Geometry: final body of the model. Coordinates: model frame, mm. A direction names the side the tool comes from. Round coordinates to 2 decimals unless told otherwise and drop trailing zeros. Loops run counter-clockwise (first coordinate to the right, second up) from the corner with the lowest first, then second, coordinate; pieces in that order, holes last. Notation, with made-up numbers: (-26, -10) - (8, -10) arc R6 ccw to (8, 1) - close; hole circle Ø1 at (80.5, 10.5). An arc over 180 degrees is marked (long way). Answer as a JSON object with one key per item and string values. Group by question number.
Item 1: Line query: line 1 (X direction, y = -0.3, z = 7.7); line 2 (Z direction, x = -6.35, y = -0.65); line 3 (Y direction, x = 1.5, z = 1.5). Output: solid intervals per line, ascending.
Item 2: Reachability of faces 5 (the face through (-6.398, 1.327, 1.357)), 6 (the face through (2.03, -6, 11)), 7 (the face through (-13, -12.55, 8)) from +Z, -Z, +X, -X, +Y, -Y: full face, straight path, thin tool, end or side. Return the list, or none.
Item 3: Section B-B (x = -6.35). Return the cut outline in (y, z).
Item 4: Section A-A (z = 4). Return the cut outline in (x, y).
Item 5: Section C-C (y = -10.75). Return the cut outline in (x, z).
Item 6: Section D-D (z = 7.7). Return the cut outline in (x, y).
Item 7: First-contact query: pin 1 (7 mm diameter, centred on x = -7, y = -3.5, fed in from -Z); pin 2 (0.7 mm diameter, centred on x = -15.5, y = -5.5, fed in from +Z); pin 3 (3.5 mm diameter, centred on y = -3, z = 5.5, fed in from -X). Flat tips, straight axial feed; report the tip coordinate or a pass-through.
Item 8: Draft query along X for faces 1 (the face through (2.03, -6, 5)), 2 (the face through (-16.245, 1.123, 0.801)), 3 (the face through (-9.243, 1.245, 14.327)), 4 (the face through (-6, 0.95, 13)). Return one class per face: released by +X, released by -X, zero draft, split by the parting line, or undercut.
Autodesk Inventor part; units mm, degrees
ref_plane "Work Plane9" through (-1.05, -12.7, 2.7) normal (0, 1, 0) x (0, 0, 1)
ref_plane "YZ Plane" through (0, 0, 0) normal (1, 0, 0) x (0, 1, 0)
ref_plane "XZ Plane" through (0, 0, 0) normal (0, 1, 0) x (-1, 0, 0)
ref_plane "Work Plane8" through (7.15, 0.8, 25.4) normal (0, 1, 0) x (1, 0, 0)
sketch "Sketch21" plane through (7.15, 0.8, 25.4) normal (0, 1, 0) x (1, 0, 0)
  line L0 (-3, 3) -> (-24, 3)
  line L1 (-3, 197) -> (-3, 3)
  line L2 (-24, 197) -> (-3, 197)
  line L3 (-24, 3) -> (-24, 197)
  line L4 (-4.819988, 19.366667) -> (-3.319988, 19.366667)
  line L5 (-3.319988, 19.366667) -> (-3.319988, 16.033333)
  line L6 (-3.319988, 16.033333) -> (-4.819988, 16.033333)
  line L7 (-4.819988, 16.033333) -> (-4.819988, 12.7)
  line L8 (-4.819988, 12.7) -> (-22.180012, 12.7)
  line L9 (-22.180012, 12.7) -> (-22.180012, 16.033333)
  line L10 (-22.180012, 16.033333) -> (-23.680012, 16.033333)
  line L11 (-23.680012, 16.033333) -> (-23.680012, 19.366667)
  line L12 (-23.680012, 19.366667) -> (-22.180012, 19.366667)
  line L13 (-22.180012, 19.366667) -> (-22.180012, 22.7)
  line L14 (-22.180012, 22.7) -> (-4.819988, 22.7)
  line L15 (-4.819988, 22.7) -> (-4.819988, 19.366667)
  line L16 (-21.880012, 22.4) -> (-21.880012, 19.066667)
  line L17 (-21.880012, 19.066667) -> (-23.380012, 19.066667)
  line L18 (-23.380012, 19.066667) -> (-23.380012, 16.333333)
  line L19 (-23.380012, 16.333333) -> (-21.880012, 16.333333)
  line L20 (-21.880012, 16.333333) -> (-21.880012, 13)
  line L21 (-21.880012, 13) -> (-5.119988, 13)
  line L22 (-5.119988, 13) -> (-5.119988, 16.333333)
  line L23 (-5.119988, 16.333333) -> (-3.619988, 16.333333)
  line L24 (-3.619988, 16.333333) -> (-3.619988, 19.066667)
  line L25 (-3.619988, 19.066667) -> (-5.119988, 19.066667)
  line L26 (-5.119988, 19.066667) -> (-5.119988, 22.4)
  line L27 (-5.119988, 22.4) -> (-21.880012, 22.4)
  point P0 (-7.15, 25.4)
  dimension "d99" = 0.3
  dimension "d100" = 0.3
  dimension "d101" = 0.3
  dimension "d102" = 0.3
  dimension "d103" = 0.3
  dimension "d104" = 0.3
  dimension "d105" = 0.3
  dimension "d106" = 0.3
  dimension "d107" = 0.3
  dimension "d108" = 0.3
  dimension "d109" = 0.3
  dimension "d110" = 0.3
ref_plane "Work Plane9" through (-1.05, -12.7, 2.7) normal (0, 1, 0) x (0, 0, 1)
sketch "Sketch21 outline for Extrusion20" plane through (7.15, 0.8, 25.4) normal (0, 1, 0) x (1, 0, 0)
  line L0 (-5.119988, 22.4) -> (-21.880012, 22.4)
  line L1 (-5.119988, 19.066667) -> (-5.119988, 22.4)
  line L2 (-3.619988, 19.066667) -> (-5.119988, 19.066667)
  line L3 (-3.619988, 16.333333) -> (-3.619988, 19.066667)
  line L4 (-5.119988, 16.333333) -> (-3.619988, 16.333333)
  line L5 (-5.119988, 13) -> (-5.119988, 16.333333)
  line L6 (-21.880012, 13) -> (-5.119988, 13)
  line L7 (-21.880012, 16.333333) -> (-21.880012, 13)
  line L8 (-23.380012, 16.333333) -> (-21.880012, 16.333333)
  line L9 (-23.380012, 19.066667) -> (-23.380012, 16.333333)
  line L10 (-21.880012, 19.066667) -> (-23.380012, 19.066667)
  line L11 (-21.880012, 22.4) -> (-21.880012, 19.066667)
extrude "Extrusion20" add sketch "Sketch21 outline for Extrusion20" against normal up to surface (13.5 mm away)
sketch "Sketch22" plane through (-14.730012, 0.8, 12.4) normal (0, 0, 1) x (1, 0, 0)
  circle A0 centre (8.380012, -13.5) radius 5 construction
  arc A1 (3.080012, -13.5) -> (13.680012, -13.5) centre (8.380012, -13.5) ccw
  arc A2 (13.680012, -13.5) -> (3.080012, -13.5) centre (8.380012, -13.5) ccw
  point P0 (14.730012, -0.8)
sketch "Sketch22 outline for Extrusion21" plane through (-14.730012, 0.8, 12.4) normal (0, 0, 1) x (1, 0, 0)
  arc A0 (13.680012, -13.5) -> (3.080012, -13.5) centre (8.380012, -13.5) ccw
  arc A1 (3.080012, -13.5) -> (13.680012, -13.5) centre (8.380012, -13.5) ccw
extrude "Extrusion21" cut sketch "Sketch22 outline for Extrusion21" against normal through all
sketch "Sketch23" plane through (7.15, 0.8, 25.4) normal (0, 1, 0) x (1, 0, 0)
  line L0 (-21.880012, 22.4) -> (-21.880012, 19.066667)
  line L1 (-21.880012, 19.066667) -> (-23.380012, 19.066667)
  line L2 (-23.380012, 19.066667) -> (-23.380012, 16.333333)
  line L3 (-23.380012, 16.333333) -> (-21.880012, 16.333333)
  line L4 (-21.880012, 16.333333) -> (-21.880012, 13)
  line L5 (-21.880012, 13) -> (-5.119988, 13)
  line L6 (-5.119988, 13) -> (-5.119988, 16.333333)
  line L7 (-5.119988, 16.333333) -> (-3.619988, 16.333333)
  line L8 (-3.619988, 16.333333) -> (-3.619988, 19.066667)
  line L9 (-3.619988, 19.066667) -> (-5.119988, 19.066667)
  line L10 (-5.119988, 19.066667) -> (-5.119988, 22.4)
  line L11 (-5.119988, 22.4) -> (-21.880012, 22.4)
  line L12 (-24, 3) -> (-24, 197)
  line L13 (-3, 197) -> (-3, 3)
  line L14 (-23.680012, 24.9) -> (-3.319988, 24.9)
  line L15 (-3.319988, 24.9) -> (-3.319988, 10.5)
  line L16 (-3.319988, 10.5) -> (-23.680012, 10.5)
  line L17 (-23.680012, 10.5) -> (-23.680012, 24.9)
  point P0 (-7.15, 25.4)
  dimension "d115" = 2.5
  dimension "d116" = 2.5
  dimension "d117" = 0.3
  dimension "d118" = 0.3
sketch "Sketch23 outline for Extrusion22" plane through (7.15, 0.8, 25.4) normal (0, 1, 0) x (1, 0, 0)
  line L0 (-23.680012, 24.9) -> (-3.319988, 24.9)
  line L1 (-3.319988, 24.9) -> (-3.319988, 10.5)
  line L2 (-3.319988, 10.5) -> (-23.680012, 10.5)
  line L3 (-23.680012, 10.5) -> (-23.680012, 24.9)
extrude "Extrusion22" add sketch "Sketch23 outline for Extrusion22" along normal blind 1.5
sketch "Sketch24" plane through (-16.530012, 0.8, 14.9) normal (0, 0, 1) x (1, 0, 0)
  line L0 (20.360025, 1.5) -> (0, 1.5)
  line L1 (0, 0) -> (0, 1.5)
  line L2 (20.360025, 0) -> (0, 0)
  line L3 (20.360025, 0) -> (20.360025, 1.5)
  line L4 (6.786675, 0) -> (13.57335, 0)
  line L5 (13.57335, 0) -> (13.57335, 0.75)
  line L6 (13.57335, 0.75) -> (6.786675, 0.75)
  line L7 (6.786675, 0.75) -> (6.786675, 0)
  point P0 (16.530012, -0.8)
  dimension "d121" = 20.36002
  dimension "d122" = 6.78667
  dimension "d123" = 6.78667
  dimension "d124" = 0.75
  dimension "d125" = 1.5
sketch "Sketch24 outline for Extrusion23" plane through (-16.530012, 0.8, 14.9) normal (0, 0, 1) x (1, 0, 0)
  line L0 (6.786675, 0.75) -> (6.786675, 0)
  line L1 (13.57335, 0.75) -> (6.786675, 0.75)
  line L2 (13.57335, 0) -> (13.57335, 0.75)
  line L3 (6.786675, 0) -> (13.57335, 0)
extrude "Extrusion23" cut sketch "Sketch24 outline for Extrusion23" against normal blind 1.5
sketch "Sketch25" plane through (3.830012, 0.8, 0.5) normal (0, 0, -1) x (-1, 0, 0)
  line L0 (6.786675, 0.75) -> (6.786675, 0)
  line L1 (13.57335, 0.75) -> (6.786675, 0.75)
  line L2 (13.57335, 0) -> (13.57335, 0.75)
  line L3 (20.360025, 0) -> (0, 0)
  point P0 (3.830012, -0.8)
fillet "Fillet13" radius 2 3 edges at (-9.7433, 1.55, 14.15) (-2.9567, 1.55, 14.15) (-6.35, 1.55, 13.4)
sketch "Sketch25 outline for Extrusion24" plane through (3.830012, 0.8, 0.5) normal (0, 0, -1) x (-1, 0, 0)
  line L0 (13.57335, 0.75) -> (6.786675, 0.75)
  line L1 (13.57335, 0) -> (13.57335, 0.75)
  line L2 (6.786675, 0) -> (13.57335, 0)
  line L3 (6.786675, 0.75) -> (6.786675, 0)
extrude "Extrusion24" cut sketch "Sketch25 outline for Extrusion24" against normal blind 1.5
fillet "Fillet14" radius 2 3 edges at (-2.9567, 1.55, 1.25) (-9.7433, 1.55, 1.25) (-6.35, 1.55, 2)
fillet "Fillet15" radius 1 8 edges at (-6.35, 2.3, 0.5) (3.83, 2.3, 7.7) (-6.35, 2.3, 14.9) (-16.53, 2.3, 7.7) (3.83, 1.55, 0.5) (3.83, 1.55, 14.9) (-16.53, 1.55, 0.5) (-16.53, 1.55, 14.9)
sketch "Sketch26" plane through (-16.230012, -12.7, 9.066667) normal (0, -1, 0) x (1, 0, 0)
  line L0 (4.580012, -6.066667) -> (4.580012, 3.333333)
  line L1 (4.580012, 3.333333) -> (1.5, 3.333333)
  line L2 (1.5, 3.333333) -> (1.5, 0)
  line L3 (1.5, 0) -> (0, 0)
  line L4 (0, 0) -> (0, -2.733333)
  line L5 (0, -2.733333) -> (1.5, -2.733333)
  line L6 (1.5, -2.733333) -> (1.5, -6.066667)
  line L7 (1.5, -6.066667) -> (4.580012, -6.066667)
  line L8 (15.180012, 3.333333) -> (15.180012, -6.066667)
  line L9 (15.180012, -6.066667) -> (18.260025, -6.066667)
  line L10 (18.260025, -6.066667) -> (18.260025, -2.733333)
  line L11 (18.260025, -2.733333) -> (19.760025, -2.733333)
  line L12 (19.760025, -2.733333) -> (19.760025, 0)
  line L13 (19.760025, 0) -> (18.260025, 0)
  line L14 (18.260025, 0) -> (18.260025, 3.333333)
  line L15 (18.260025, 3.333333) -> (15.180012, 3.333333)
  point P0 (16.230012, -9.066667)
sketch "Sketch26 outline for Extrusion25" plane through (-16.230012, -12.7, 9.066667) normal (0, -1, 0) x (1, 0, 0)
  line L0 (1.5, -6.066667) -> (4.580012, -6.066667)
  line L1 (1.5, -2.733333) -> (1.5, -6.066667)
  line L2 (0, -2.733333) -> (1.5, -2.733333)
  line L3 (0, 0) -> (0, -2.733333)
  line L4 (1.5, 0) -> (0, 0)
  line L5 (1.5, 3.333333) -> (1.5, 0)
  line L6 (4.580012, 3.333333) -> (1.5, 3.333333)
  line L7 (4.580012, -6.066667) -> (4.580012, 3.333333)
  line L8 (18.260025, 3.333333) -> (15.180012, 3.333333)
  line L9 (18.260025, 0) -> (18.260025, 3.333333)
  line L10 (19.760025, 0) -> (18.260025, 0)
  line L11 (19.760025, -2.733333) -> (19.760025, 0)
  line L12 (18.260025, -2.733333) -> (19.760025, -2.733333)
  line L13 (18.260025, -6.066667) -> (18.260025, -2.733333)
  line L14 (15.180012, -6.066667) -> (18.260025, -6.066667)
  line L15 (15.180012, 3.333333) -> (15.180012, -6.066667)
extrude "Extrusion25" cut sketch "Sketch26 outline for Extrusion25" against normal blind 0.15
sketch "Sketch27" plane through (7.15, 0.8, 25.4) normal (0, -1, 0) x (1, 0, 0)
  line L0 (-3.619988, -16.333333) -> (-3.619988, -19.066667)
  line L1 (-3.619988, -19.066667) -> (-5.119988, -19.066667)
  line L2 (-5.119988, -19.066667) -> (-5.119988, -22.4)
  line L3 (-5.119988, -22.4) -> (-21.880012, -22.4)
  line L4 (-21.880012, -22.4) -> (-21.880012, -19.066667)
  line L5 (-21.880012, -19.066667) -> (-23.380012, -19.066667)
  line L6 (-23.380012, -19.066667) -> (-23.380012, -16.333333)
  line L7 (-23.380012, -16.333333) -> (-21.880012, -16.333333)
  line L8 (-21.880012, -16.333333) -> (-21.880012, -13)
  line L9 (-21.880012, -13) -> (-5.119988, -13)
  line L10 (-5.119988, -13) -> (-5.119988, -16.333333)
  line L11 (-5.119988, -16.333333) -> (-3.619988, -16.333333)
  arc A0 (-22.680012, -10.5) -> (-23.680012, -11.5) centre (-22.680012, -11.5) ccw
  line L12 (-23.680012, -11.5) -> (-23.680012, -23.9)
  arc A1 (-23.680012, -23.9) -> (-22.680012, -24.9) centre (-22.680012, -23.9) ccw
  line L13 (-22.680012, -24.9) -> (-16.893337, -24.9)
  line L14 (-16.893337, -24.9) -> (-16.893337, -23.4)
  line L15 (-16.893337, -23.4) -> (-10.106663, -23.4)
  line L16 (-10.106663, -23.4) -> (-10.106663, -24.9)
  line L17 (-10.106663, -24.9) -> (-4.319988, -24.9)
  arc A2 (-4.319988, -24.9) -> (-3.319988, -23.9) centre (-4.319988, -23.9) ccw
  line L18 (-3.319988, -23.9) -> (-3.319988, -11.5)
  arc A3 (-3.319988, -11.5) -> (-4.319988, -10.5) centre (-4.319988, -11.5) ccw
  line L19 (-4.319988, -10.5) -> (-10.106663, -10.5)
  line L20 (-10.106663, -10.5) -> (-10.106663, -12)
  line L21 (-10.106663, -12) -> (-16.893337, -12)
  line L22 (-16.893337, -12) -> (-16.893337, -10.5)
  line L23 (-16.893337, -10.5) -> (-22.680012, -10.5)
  point P0 (-7.15, -25.4)
sketch "Sketch27 outline for Extrusion26" plane through (7.15, 0.8, 25.4) normal (0, -1, 0) x (1, 0, 0)
  line L0 (-16.893337, -10.5) -> (-22.680012, -10.5)
  line L1 (-16.893337, -12) -> (-16.893337, -10.5)
  arc A0 (-22.680012, -10.5) -> (-23.680012, -11.5) centre (-22.680012, -11.5) ccw
  line L2 (-10.106663, -12) -> (-16.893337, -12)
  line L3 (-23.680012, -11.5) -> (-23.680012, -23.9)
  line L4 (-10.106663, -10.5) -> (-10.106663, -12)
  arc A1 (-23.680012, -23.9) -> (-22.680012, -24.9) centre (-22.680012, -23.9) ccw
  line L5 (-4.319988, -10.5) -> (-10.106663, -10.5)
  line L6 (-22.680012, -24.9) -> (-16.893337, -24.9)
  arc A2 (-3.319988, -11.5) -> (-4.319988, -10.5) centre (-4.319988, -11.5) ccw
  line L7 (-16.893337, -24.9) -> (-16.893337, -23.4)
  line L8 (-3.319988, -23.9) -> (-3.319988, -11.5)
  line L9 (-16.893337, -23.4) -> (-10.106663, -23.4)
  arc A3 (-4.319988, -24.9) -> (-3.319988, -23.9) centre (-4.319988, -23.9) ccw
  line L10 (-10.106663, -23.4) -> (-10.106663, -24.9)
  line L11 (-10.106663, -24.9) -> (-4.319988, -24.9)
  line L12 (-5.119988, -16.333333) -> (-3.619988, -16.333333)
  line L13 (-5.119988, -13) -> (-5.119988, -16.333333)
  line L14 (-21.880012, -13) -> (-5.119988, -13)
  line L15 (-21.880012, -16.333333) -> (-21.880012, -13)
  line L16 (-23.380012, -16.333333) -> (-21.880012, -16.333333)
  line L17 (-23.380012, -19.066667) -> (-23.380012, -16.333333)
  line L18 (-21.880012, -19.066667) -> (-23.380012, -19.066667)
  line L19 (-21.880012, -22.4) -> (-21.880012, -19.066667)
  line L20 (-5.119988, -22.4) -> (-21.880012, -22.4)
  line L21 (-5.119988, -19.066667) -> (-5.119988, -22.4)
  line L22 (-3.619988, -19.066667) -> (-5.119988, -19.066667)
  line L23 (-3.619988, -16.333333) -> (-3.619988, -19.066667)
extrude "Extrusion26" cut sketch "Sketch27 outline for Extrusion26" against normal blind 0.15
sketch "Sketch28" plane through (7.15, 2.3, 25.4) normal (0, 1, 0) x (1, 0, 0)
  circle A0 centre (-13.5, 17.7) radius 2
  point P0 (-7.15, 25.4)
sketch "Sketch28 outline for Extrusion27" plane through (7.15, 2.3, 25.4) normal (0, 1, 0) x (1, 0, 0)
  circle A0 centre (-13.5, 17.7) radius 2
extrude "Extrusion27" cut sketch "Sketch28 outline for Extrusion27" against normal blind 5
equation "\"d100\" = d99"
equation "\"d101\" = d99"
equation "\"d102\" = d101"
equation "\"d103\" = d102"
equation "\"d104\" = d102"
equation "\"d105\" = d104"
equation "\"d106\" = d105"
equation "\"d107\" = d106"
equation "\"d108\" = d106"
equation "\"d109\" = d107"
equation "\"d110\" = d109"
equation "\"d116\" = d115"
equation "\"d118\" = d117"
equation "\"d122\" = 0.333333 * d121"
equation "\"d123\" = d122"
equation "\"d124\" = 0.5 * d125"
properties part number "InternalKey"
Values:
{
 "1": {"line 1": "x = -16.23 to -8.35, -4.35 to 3.53", "line 2": "z = 3 to 5.7, 9.7 to 12.4", "line 3": "y = 0.95 to 2.3"},
 "2": {"face 5": "-Z, -Y", "face 6": "+Z, +X, -Y", "face 7": "+Z, -Z, -X, -Y"},
 "3": {"outline": "(-7.4, 3) - (0.95, 3) - (0.95, 2) - (0.8, 2) arc R2 cw to (1.55, 0.53) arc R1 ccw to (2.3, 1.5) - (2.3, 5.7) - (-2.7, 5.7) - (-2.7, 9.7) - (2.3, 9.7) - (2.3, 13.9) arc R1 ccw to (1.55, 14.87) arc R2 cw to (0.8, 13.4) - (0.95, 13.4) - (0.95, 12.4) - (-7.4, 12.4) - close"},
 "4": {"outline": "(-16.53, 0.95) - (-14.73, 0.95) - (-14.73, -12.55) - (-11.65, -12.55) - (-11.65, -12.7) arc R5.3 cw to (-1.05, -12.7) - (-1.05, -12.55) - (2.03, -12.55) - (2.03, 0.95) - (3.83, 0.95) - (3.83, 1.3) arc R1 ccw to (2.83, 2.3) - (-15.53, 2.3) arc R1 ccw to (-16.53, 1.3) - close"},
 "5": {"outline": "(-16.23, 6.33) - (-14.73, 6.33) - (-14.73, 3) - (-11.28, 3) - (-11.28, 12.4) - (-14.73, 12.4) - (-14.73, 9.07) - (-16.23, 9.07) - close; (-1.42, 3) - (2.03, 3) - (2.03, 6.33) - (3.53, 6.33) - (3.53, 9.07) - (2.03, 9.07) - (2.03, 12.4) - (-1.42, 12.4) - close"},
 "6": {"outline": "(-16.53, 0.95) - (-16.23, 0.95) - (-16.23, -12.55) - (-11.65, -12.55) - (-11.65, -12.7) arc R5.3 cw to (-1.05, -12.7) - (-1.05, -12.55) - (3.53, -12.55) - (3.53, 0.95) - (3.83, 0.95) - (3.83, 1.3) arc R1 ccw to (2.83, 2.3) - (-4.35, 2.3) - (-4.35, -2.7) - (-8.35, -2.7) - (-8.35, 2.3) - (-15.53, 2.3) arc R1 ccw to (-16.53, 1.3) - close"},
 "7": {"pin 1": "stops at z = 3", "pin 2": "stops at z = 9.07", "pin 3": "stops at x = -16.23"},
 "8": {"face 1": "released by +X", "face 2": "released by -X", "face 3": "undercut", "face 4": "zero draft"}
}
